Source: CAD feature listing. Evaluate the final solid. Frame: model axes, mm. Coordinates: 2 decimals unless noted, no trailing zeros. Order: outer loops, then holes, each group sorted by start corner. A loop starts at its lowest first (then second) coordinate and runs counter-clockwise, first axis right, second up. Notation, with made-up numbers: (87.25, 76) -> (109.25, 76) arc R14 cw to (109.25, 100) -> close; hole circle Ø8 at (63.25, -35.75). An arc over 180 degrees is marked (long way). Write each question's results on one line, items separated by ' | '. Start each with the question number.
from build123d import *

# Parameters (mm, degrees)
SKETCH1_R               = 19.05
BOSS_EXTRUDE1_DEPTH     = 25.4
CUT_EXTRUDE1_DEPTH      = 36.83
CUT_EXTRUDE1_DEPTH_BACK = 7.366
SKETCH3_R               = 2.54


with BuildPart() as part:
    # Sketch1 → Boss-Extrude1 (new body)
    with BuildSketch(Plane.XY):
        Circle(SKETCH1_R)
    extrude(amount=BOSS_EXTRUDE1_DEPTH)

    # Sketch2 → Cut-Revolve1 (revolve, cut)
    with BuildSketch(Plane(origin=(0, 0, 0), x_dir=(0, 0, -1), z_dir=(1, 0, 0)), mode=Mode.PRIVATE) as cut_revolve1_sk:
        with BuildLine():
            Line((-3.81, 19.05), (-21.59, 19.05))
            ThreePointArc((-21.59, 19.05), (-12.7, 5.130913707), (-3.81, 19.05))
        make_face()
    revolve(cut_revolve1_sk.sketch.rotate(Axis((0, 0, 36.401990555), (0, 0, -1)), 90), axis=Axis((0, 0, 36.401990555), (0, 0, -1)), mode=Mode.SUBTRACT)

    # Sketch3 → Cut-Extrude1 (cut, two sides: drawn at the far end of the back side and taken through both)
    with BuildSketch(Plane.XY.offset(-CUT_EXTRUDE1_DEPTH_BACK)):
        Circle(SKETCH3_R)
    extrude(amount=CUT_EXTRUDE1_DEPTH + CUT_EXTRUDE1_DEPTH_BACK, mode=Mode.SUBTRACT)


solid = part.part
(1) Section D-D on z = 14. Return the cut outline in (x, y), then the cut area to 3 significant figures.
(2) First-contact query: P1, Ø6, axis at y = 0, z = 13.5, coming from the +X side; P2, Ø12, axis at x = 11, z = 3.5, coming from the -Y side; P3, Ø6, axis at x = 8, z = 8.5, coming from the -Y side. Flat tips, straight axial feed; report the tip coordinate or a pass-through.
(3) Draft query along X for faces 1 (the cylindrical face through (-0.33, 2.52, 12.52)), 2 (the cylindrical face through (-15.12, -11.59, 1.88)), 3 (the flat face through (4, 0, 0)). Return one class per face: released by +X, released by -X, zero draft, split by the parting line, or undercut.
(4) Section C-C on z = 19.75. Return the cut outline in (x, y).
(5) Line query: L1, parallel to Z at x = 14.5, y = -2; L2, parallel to Y at x = 0, z = 6.75; L3, parallel to Z at x = -12, y = -11. Output: solid intervals per line, ascending.
(6) Section A-A on x = 0. Return the cut outline in (y, z).
Results list:
1) outline: circle Ø10.44 at (0, 0); hole circle Ø5.08 at (0, 0) | area: 65.3 mm²
2) P1: stops at x = 5.9 | P2: stops at y = -18.38 | P3: stops at y = -4.57
3) face 1: undercut | face 2: split by the parting line | face 3: zero draft
4) outline: circle Ø16.25 at (0, 0); hole circle Ø5.08 at (0, 0)
5) L1: z = 0 to 2.91, 22.49 to 25.4 | L2: y = -7.14 to -2.54, 2.54 to 7.14 | L3: z = 0 to 2.99, 22.41 to 25.4
6) outline: (-19.05, 0) -> (-2.54, 0) -> (-2.54, 25.4) -> (-19.05, 25.4) -> (-19.05, 21.59) arc R9.8 cw (long way) to (-19.05, 3.81) -> close; (2.54, 0) -> (19.05, 0) -> (19.05, 3.81) arc R9.8 cw (long way) to (19.05, 21.59) -> (19.05, 25.4) -> (2.54, 25.4) -> close
